Geometry check sheet. Reference: the model listing, model coordinates, mm. Coordinates: 2 decimals unless noted, no trailing zeros. Write each loop counter-clockwise with the first axis right and the second up, starting at its lowest first coordinate (ties: lowest second). Pieces come first, ordered by that corner, then holes. Notation, with made-up numbers: (-12.5, 2) -> (-8.5, 2) arc R24 cw to (-8.5, 22) -> close; hole circle Ø3 at (-17, 35). An arc over 180 degrees is marked (long way). Answer as CSV lines item,"result".
Autodesk Inventor part; units mm, degrees
ref_plane "YZ Plane" through (0, 0, 0) normal (1, 0, 0) x (0, 1, 0)
ref_plane "XZ Plane" through (0, 0, 0) normal (0, 1, 0) x (-1, 0, 0)
ref_plane "XY Plane" through (0, 0, 0) normal (0, 0, 1) x (1, 0, 0)
sketch "Sketch1" plane through (0, 0, 0) normal (0, 1, 0) x (-1, 0, 0)
  point P0 (0, 0)
sketch "Sketch3" plane through (0, 0, 0) normal (0, 1, 0) x (-1, 0, 0)
  line L0 (113.8824, -237.8336) -> (98.8824, -237.8336)
  line L1 (128.8824, -242.8336) -> (113.8824, -242.8336)
  line L2 (128.8824, -242.8336) -> (128.8824, -237.8336)
  line L3 (98.8824, -237.8336) -> (98.8824, -242.8336)
  line L4 (113.8824, -242.8336) -> (113.8824, -237.8336)
  line L5 (48.8824, -156.8908) -> (45.8824, -156.8908)
  line L6 (48.8824, -156.8908) -> (48.8824, -112.2516)
  line L7 (48.8824, -112.2516) -> (45.8824, -112.2516)
  line L8 (45.8824, -112.2516) -> (45.8824, -65.4156)
  line L9 (48.8824, -65.4156) -> (45.8824, -65.4156)
  line L10 (48.8824, -156.8908) -> (48.8824, -112.2516)
  line L11 (98.8824, -242.8336) -> (78.8824, -242.8336)
  line L12 (63.8824, -237.8336) -> (75.0605, -237.8336)
  line L13 (48.8824, -237.8336) -> (48.8824, -202.2369)
  line L14 (48.8824, -202.2369) -> (45.8824, -202.2369)
  line L15 (45.8824, -202.2369) -> (45.8824, -156.8908)
  line L16 (48.8824, -20.7764) -> (45.8824, -20.7764)
  line L17 (45.8824, -20.7764) -> (45.8824, 24.5697)
  line L18 (48.8824, -65.4156) -> (48.8824, -20.7764)
  line L19 (48.8824, -65.4156) -> (48.8824, -20.7764)
  line L20 (48.8824, 24.5697) -> (45.8824, 24.5697)
  line L21 (113.8824, 65.1664) -> (113.8824, 62.1664)
  line L22 (48.8824, 24.5697) -> (48.8824, 62.1664)
  line L23 (48.8824, 24.5697) -> (48.8824, 65.1664)
  line L24 (48.8824, 65.1664) -> (63.8824, 65.1664)
  line L25 (63.8824, 62.1664) -> (78.8824, 62.1664)
  line L26 (63.8824, 65.1664) -> (63.8824, 62.1664)
  line L27 (78.8824, 62.1664) -> (78.8824, 65.1664)
  line L28 (78.8824, 65.1664) -> (98.8824, 65.1664)
  line L29 (98.8824, 62.1664) -> (98.8824, 65.1664)
  line L30 (98.8824, 62.1664) -> (113.8824, 62.1664)
  line L31 (128.8824, 62.1664) -> (128.8824, 65.1664)
  line L32 (113.8824, 65.1664) -> (128.8824, 65.1664)
  line L33 (63.8824, -237.8336) -> (78.8824, -237.8336)
  line L34 (48.8824, -242.8336) -> (48.8824, -237.8336)
  line L35 (48.8824, -242.8336) -> (63.8824, -242.8336)
  line L36 (63.8824, -242.8336) -> (63.8824, -237.8336)
  line L37 (78.8824, -237.8336) -> (78.8824, -242.8336)
  line L38 (78.8824, -237.8336) -> (63.8824, -237.8336)
  line L39 (171.6524, -88.8336) -> (171.6524, -237.8336)
  line L40 (171.6524, -237.8336) -> (128.8824, -237.8336)
  line L41 (171.6524, -88.8336) -> (171.6524, 62.1664)
  line L42 (171.6524, 62.1664) -> (128.8824, 62.1664)
  point P0 (0, 0)
  point P1 (0, 0)
  point P2 (106.3824, -237.8336)
  point P3 (47.3824, -202.2369)
  point P4 (0, 0)
  point P5 (106.3824, 62.1664)
  point P6 (121.3824, 65.1664)
  dimension "d54" = 80
  dimension "d55" = 15
  dimension "d56" = 15
  dimension "d57" = 300
  dimension "d58" = 3
  dimension "d59" = 5
  dimension "d60" = 44.6392
  dimension "d61" = 37.5967
  dimension "d62" = 44.6392
  dimension "d63" = 40.5967
  dimension "d64" = 45.3461
  dimension "d66" = 45.3461
  dimension "d67" = 20
  dimension "d68" = 15
  dimension "d69" = 15
  dimension "d70" = 15
  dimension "d71" = 15
  dimension "d72" = 15
  dimension "d73" = 15
  dimension "d74" = 20
  dimension "d75" = 308
extrude "Extrusion2" add sketch "Sketch3" along normal blind 3
properties part number "mieng_ben_3mm"
Item 1: Thickness scan on probe 1 along Z at (x, y) = (-158.5, 0.6); probe 2 along X at (y, z) = (1.4, -22). Record the ranges inside material, lowest first.
Responses:
probe 1,"z = -237.83 to 62.17"
probe 2,"x = -171.65 to -48.88"
Item 2: Depth check by flat-ended pin: pin 1 Ø0.9 at (y, z) = (1, 63.5) entering from -X; pin 2 Ø1.5 at (x, y) = (-73.5, 1) entering from -Z; pin 3 Ø1.5 at (x, y) = (-48, 2) entering from +Z; pin 4 Ø8 at (x, z) = (-111.5, -79) entering from -Y. Enter the tip coordinate at first touch or a pass-through.
Responses:
pin 1,"stops at x = -128.88"
pin 2,"stops at z = -237.83"
pin 3,"stops at z = 24.57"
pin 4,"stops at y = 0"
Item 3: Cross-section at B-B, the plane z = 31.5. Record the cut outline in (x, y).
Responses:
outline,"(-171.65, 0) -> (-48.88, 0) -> (-48.88, 3) -> (-171.65, 3) -> close"
Item 4: Cross-section at A-A, the plane x = -141. Record the cut outline in (y, z), plus the area to 3 significant figures.
Responses:
outline,"(0, -237.83) -> (3, -237.83) -> (3, 62.17) -> (0, 62.17) -> close"
area,"900 mm2"
